Drawing for the job (mm, zero at the part's lowest x, y, z). Coordinates: 2 decimals unless noted, no trailing zeros. Order: outer loops, then holes, each group sorted by start corner. A loop starts at its lowest first (then second) coordinate and runs counter-clockwise, first axis right, second up. Notation, with made-up numbers: (6.5, 20) - (45.5, 20) arc R13 cw to (45.5, 35) - close; hole circle Ø7 at (64, -33). An arc over 180 degrees is marked (long way). Put each result on its own line as item: value. Start each with the question number.
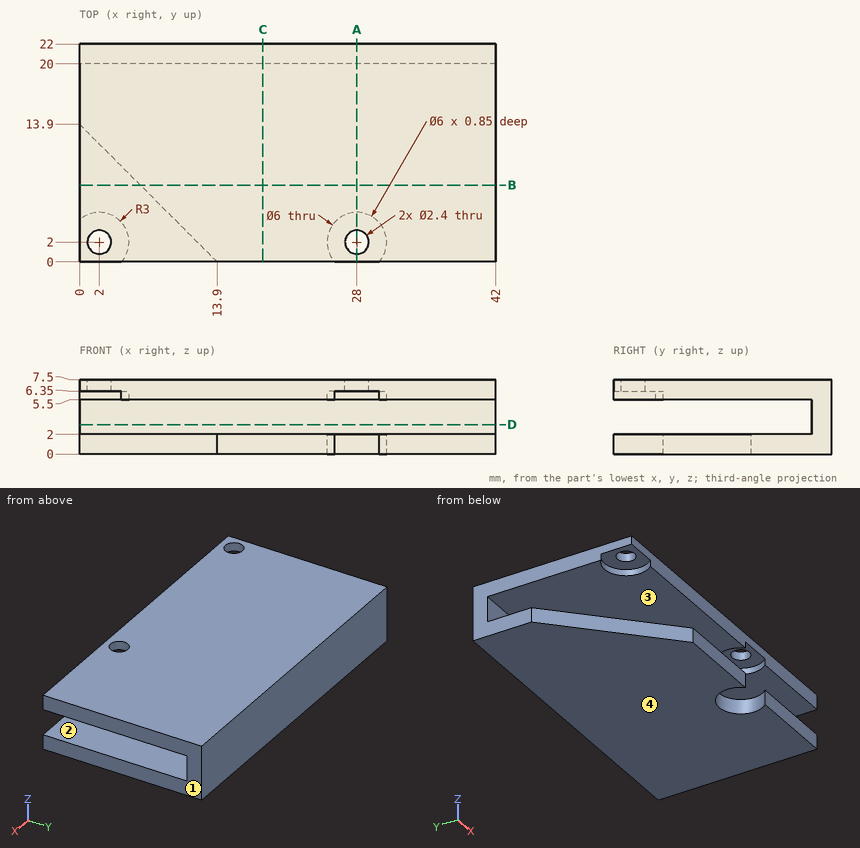
Item 1: Pull direction Z, two halves, no side cores. Call the marked faces 1, 2, 3 and 4: pulls with the +Z half, pulls with the -Z half, needs draft (parallel to the pull), parting line crosses it, or undercut.
Item 2: Wall check: line 1 along X through (y, z) = (2, 6.95); line 2 along Z through (x, y) = (15.5, 16.75); line 3 along Y through (x, z) = (31.5, 4.5). Give the ranges that are in metal, low to high.
Item 3: Slice it at C-C, the plane x = 18.5. Give the cut face in (y, z).
Item 4: Slice it at A-A, the plane x = 28. Give the cut face in (y, z).
Item 5: Slice it at D-D, the plane z = 3. Give the cut face in (x, y).
Item 6: Slice it at B-B, the plane y = 7.75. Give the cut face in (x, z), plus the area to 3 significant figures.
Item 7: Flat gauge pins, fed straight in: pin 1 Ø12 at (x, y) = (13, 12.5) entering from -Z; pin 2 Ø2.5 at (x, y) = (2, 1.5) entering from -Z; pin 3 Ø1.9 at (x, y) = (28, 2) entering from +Z. Where does each tip first touch, or does it go through?
Here are the results:
1. face 1: needs draft
1. face 2: undercut
1. face 3: undercut
1. face 4: pulls with the -Z half
2. line 1: x = 0 to 0.8, 3.2 to 26.8, 29.2 to 42
2. line 2: z = 0 to 2, 5.5 to 7.5
2. line 3: y = 20 to 22
3. outline: (0, 0) - (22, 0) - (22, 7.5) - (0, 7.5) - (0, 5.5) - (20, 5.5) - (20, 2) - (0, 2) - close
4. outline: (0, 6.35) - (0.8, 6.35) - (0.8, 7.5) - (0, 7.5) - close; (3.2, 6.35) - (5, 6.35) - (5, 5.5) - (20, 5.5) - (20, 2) - (5, 2) - (5, 0) - (22, 0) - (22, 7.5) - (3.2, 7.5) - close
5. outline: (0, 20) - (42, 20) - (42, 22) - (0, 22) - close
6. outline: (0, 5.5) - (42, 5.5) - (42, 7.5) - (0, 7.5) - close; (6.15, 0) - (42, 0) - (42, 2) - (6.15, 2) - close
6. area: 156 mm^2
7. pin 1: stops at z = 0
7. pin 2: stops at z = 6.35
7. pin 3: passes through
